```python
from build123d import *

# Parameters (mm, degrees)
SKETCH1_W              = 220
SKETCH1_H              = 225
BOSS_EXTRUDE1_DEPTH    = 16
CUT_EXTRUDE1_REACH     = 160.153
SKETCH2_R              = 4
CUT_EXTRUDE2_REACH     = 160.153
SKETCH3_W              = 12
SKETCH3_H              = 11.5
SKETCH4_R              = 8.5
CUT_EXTRUDE3_DEPTH     = 5
M10_TAPPED_HOLE2_D     = 8.5
M10_TAPPED_HOLE3_D     = 8.5
M10_TAPPED_HOLE4_D     = 8.5
CUT_EXTRUDE4_REACH     = 160.153
CUT_EXTRUDE6_REACH     = 160.153
F_10_0MM_DOWEL_HOLE1_D = 10
CUT_EXTRUDE7_REACH     = 160.153
SKETCH34_R             = 5


with BuildPart() as part:
    # Sketch1 → Boss-Extrude1 (new body)
    with BuildSketch(Plane(origin=(0, 0, 0), x_dir=(1, 0, 0), z_dir=(0, 1, 0))):
        Rectangle(SKETCH1_W, SKETCH1_H)
    extrude(amount=-BOSS_EXTRUDE1_DEPTH)

    # Sketch2 → Cut-Extrude1 (cut, up to next)
    with BuildSketch(Plane(origin=(0, 0, 0), x_dir=(1, 0, 0), z_dir=(0, 1, 0)), mode=Mode.PRIVATE) as cut_extrude1_sk1:
        with Locations(Location((-21.75, 10.23, 0), (0, 0, 270))):
            Circle(SKETCH2_R)
    cut_extrude1_tool1 = extrude(cut_extrude1_sk1.sketch, amount=-CUT_EXTRUDE1_REACH, mode=Mode.PRIVATE) & part.part
    add(cut_extrude1_tool1.solids().sort_by_distance((-21.75, 0, -10.23))[0], mode=Mode.SUBTRACT)

    # Sketch3 → Cut-Extrude2 (cut, up to next)
    with BuildSketch(Plane.XZ.offset(16), mode=Mode.PRIVATE) as cut_extrude2_sk1:
        with BuildLine():
            Line((-77.87, 101), (-67.87, 101))
            ThreePointArc((-67.87, 101), (-67.162893219, 101.292893219), (-66.87, 102))
            Line((-66.87, 102), (-66.87, 112.5))
            Line((-66.87, 112.5), (-78.87, 112.5))
            Line((-78.87, 112.5), (-78.87, 102))
            ThreePointArc((-78.87, 102), (-78.577106781, 101.292893219), (-77.87, 101))
        make_face()
    cut_extrude2_tool1 = extrude(cut_extrude2_sk1.sketch, amount=-CUT_EXTRUDE2_REACH, mode=Mode.PRIVATE) & part.part
    # Sketch3 → Cut-Extrude2 (cut, up to next)
    with BuildSketch(Plane.XZ.offset(16), mode=Mode.PRIVATE) as cut_extrude2_sk2:
        with Locations((3.38, 106.75)):
            Rectangle(SKETCH3_W, SKETCH3_H)
    cut_extrude2_tool2 = extrude(cut_extrude2_sk2.sketch, amount=-CUT_EXTRUDE2_REACH, mode=Mode.PRIVATE) & part.part
    add(cut_extrude2_tool1.solids().sort_by_distance((-72.87, -16, 106.767242))[0], mode=Mode.SUBTRACT)
    add(cut_extrude2_tool2.solids().sort_by_distance((3.38, -16, 106.75))[0], mode=Mode.SUBTRACT)

    # Sketch4 → Cut-Extrude3 (cut)
    with BuildSketch(Plane.XZ.offset(16)):
        with Locations(Location((-35, 100, 0), (0, 0, 270))):
            Circle(SKETCH4_R)
        with Locations(Location((25, 100, 0), (0, 0, 270))):
            Circle(SKETCH4_R)
        with Locations(Location((70, 100, 0), (0, 0, 270))):
            Circle(SKETCH4_R)
        with Locations(Location((-35, -100, 0), (0, 0, 270))):
            Circle(SKETCH4_R)
        with Locations(Location((25, -100, 0), (0, 0, 270))):
            Circle(SKETCH4_R)
        with Locations(Location((70, -100, 0), (0, 0, 270))):
            Circle(SKETCH4_R)
    extrude(amount=-CUT_EXTRUDE3_DEPTH, mode=Mode.SUBTRACT)

    # M10 Tapped Hole2 (through all)
    with Locations(Plane(origin=(0, 0, 0), x_dir=(1, 0, 0), z_dir=(0, 1, 0))):
        with Locations((-95, -67.5), (-95, -37.5), (-95, 0), (-95, 37.5), (-95, 67.5), (95, 67.5), (95, 37.5), (95, 0), (95, -37.5), (95, -67.5)):
            Hole(M10_TAPPED_HOLE2_D / 2)

    # M10 Tapped Hole3 (through all)
    with Locations(Plane(origin=(0, 0, 0), x_dir=(1, 0, 0), z_dir=(0, 1, 0))):
        with Locations((-56, 92.5), (-5, 92.5), (47.5, 92.5)):
            Hole(M10_TAPPED_HOLE3_D / 2)

    # M10 Tapped Hole4 (through all)
    with Locations(Plane(origin=(0, 0, 0), x_dir=(1, 0, 0), z_dir=(0, 1, 0))):
        with Locations((-13, -90.5), (47.5, -90.5), (-56, -90.5)):
            Hole(M10_TAPPED_HOLE4_D / 2)

    # Sketch24 → Cut-Extrude4 (cut, up to next)
    with BuildSketch(Plane(origin=(0, 0, 0), x_dir=(1, 0, 0), z_dir=(0, 1, 0)), mode=Mode.PRIVATE) as cut_extrude4_sk1:
        with BuildLine():
            Line((2.25, -35.27), (2.25, -71.53))
            ThreePointArc((2.25, -71.53), (1.371320344, -73.651320344), (-0.75, -74.53))
            Line((-0.75, -74.53), (-42.75, -74.53))
            ThreePointArc((-42.75, -74.53), (-44.871320344, -73.651320344), (-45.75, -71.53))
            Line((-45.75, -71.53), (-45.75, -35.27))
            ThreePointArc((-45.75, -35.27), (-44.871320344, -33.148679656), (-42.75, -32.27))
            Line((-42.75, -32.27), (-40.75, -32.27))
            Line((-40.75, -32.27), (-40.75, -38.4))
            ThreePointArc((-40.75, -38.4), (-38.992640687, -42.642640687), (-34.75, -44.4))
            Line((-34.75, -44.4), (-30.75, -44.4))
            ThreePointArc((-30.75, -44.4), (-28.628679656, -45.278679656), (-27.75, -47.4))
            Line((-27.75, -47.4), (-27.75, -63.53))
            ThreePointArc((-27.75, -63.53), (-21.75, -69.53), (-15.75, -63.53))
            Line((-15.75, -63.53), (-15.75, -47.4))
            ThreePointArc((-15.75, -47.4), (-14.871320344, -45.278679656), (-12.75, -44.4))
            Line((-12.75, -44.4), (-8.75, -44.4))
            ThreePointArc((-8.75, -44.4), (-4.507359313, -42.642640687), (-2.75, -38.4))
            Line((-2.75, -38.4), (-2.75, -32.27))
            Line((-2.75, -32.27), (-0.75, -32.27))
            ThreePointArc((-0.75, -32.27), (1.371320344, -33.148679656), (2.25, -35.27))
        make_face()
    cut_extrude4_tool1 = extrude(cut_extrude4_sk1.sketch, amount=-CUT_EXTRUDE4_REACH, mode=Mode.PRIVATE) & part.part
    add(cut_extrude4_tool1.solids().sort_by_distance((-15.110476, 0, 55.465))[0], mode=Mode.SUBTRACT)

    # Sketch29 → Cut-Extrude6 (cut, up to next)
    with BuildSketch(Plane.XZ.offset(16), mode=Mode.PRIVATE) as cut_extrude6_sk1:
        with BuildLine():
            Line((-2.75, -47.73), (-0.75, -47.73))
            ThreePointArc((-0.75, -47.73), (1.371320344, -48.608679656), (2.25, -50.73))
            Line((2.25, -50.73), (2.25, -71.53))
            ThreePointArc((2.25, -71.53), (1.371320344, -73.651320344), (-0.75, -74.53))
            Line((-0.75, -74.53), (-42.75, -74.53))
            ThreePointArc((-42.75, -74.53), (-44.871320344, -73.651320344), (-45.75, -71.53))
            Line((-45.75, -71.53), (-45.75, -50.73))
            ThreePointArc((-45.75, -50.73), (-44.871320344, -48.608679656), (-42.75, -47.73))
            Line((-42.75, -47.73), (-40.75, -47.73))
            Line((-40.75, -47.73), (-40.75, -69.53))
            Line((-40.75, -69.53), (-2.75, -69.53))
            Line((-2.75, -69.53), (-2.75, -47.73))
        make_face()
    cut_extrude6_tool1 = extrude(cut_extrude6_sk1.sketch, amount=-CUT_EXTRUDE6_REACH, mode=Mode.PRIVATE) & part.part
    add(cut_extrude6_tool1.solids().sort_by_distance((-1.75, -16, -48.279749))[0], mode=Mode.SUBTRACT)

    # Ø10.0mm Dowel Hole1 (through all)
    with Locations(Plane(origin=(0, 0, 0), x_dir=(1, 0, 0), z_dir=(0, 1, 0))):
        with Locations((54.5, -63.53), (67.5, -38.4), (41.5, -38.4), (19.38, 26.73), (19.38, -6.27)):
            Hole(F_10_0MM_DOWEL_HOLE1_D / 2)

    # Sketch34 → Cut-Extrude7 (cut, up to next)
    with BuildSketch(Plane(origin=(0, 0, 0), x_dir=(1, 0, 0), z_dir=(0, 1, 0)), mode=Mode.PRIVATE) as cut_extrude7_sk1:
        with Locations(Location((54.5, 10.23, 0), (0, 0, 270))):
            Circle(SKETCH34_R)
    cut_extrude7_tool1 = extrude(cut_extrude7_sk1.sketch, amount=-CUT_EXTRUDE7_REACH, mode=Mode.PRIVATE) & part.part
    add(cut_extrude7_tool1.solids().sort_by_distance((54.5, 0, -10.23))[0], mode=Mode.SUBTRACT)

    # Cut-Sweep1: sweep along a curve in space
    with BuildLine() as cut_sweep1_path:
        ThreePointArc((54.5, 0, -5.23), (58.035533906, 0, -6.694466094), (59.5, 0, -10.23))
        ThreePointArc((59.5, 0, -10.23), (58.035533906, 0, -13.765533906), (54.5, 0, -15.23))
        ThreePointArc((54.5, 0, -15.23), (50.964466094, 0, -13.765533906), (49.5, 0, -10.23))
        ThreePointArc((49.5, 0, -10.23), (50.964466094, 0, -6.694466094), (54.5, 0, -5.23))
    # Sketch35 → Cut-Sweep1 (sweep, cut)
    with BuildSketch(Plane.XY.offset(-10.23)):
        Polygon((59.5, -10), (60.024077793, 0), (59.5, 0), align=None)
    sweep(path=cut_sweep1_path.line, mode=Mode.SUBTRACT)


solid = part.part
```
Design review of the part built by this model. Coordinates are the model's own, in mm. A direction names the side the tool comes from. Coordinates: 2 decimals unless noted, no trailing zeros. Loops run counter-clockwise (first coordinate to the right, second up) from the corner with the lowest first, then second, coordinate; pieces in that order, holes last.
Q1. We need section D-D on y = -2.5. State how many separate pieces and enclosed holes the cut face has, and give its area (3 significant figures).
Reported:
separate pieces: 1
enclosed holes: 25
area: 46,000 mm2
Q2. We need section B-B on z = -37.5. State the section outline as (x, y) points.
Reported:
outline: (-110, -16) - (-99.25, -16) - (-99.25, 0) - (-110, 0) - close; (-90.75, -16) - (90.75, -16) - (90.75, 0) - (-90.75, 0) - close; (99.25, -16) - (110, -16) - (110, 0) - (99.25, 0) - close
Q3. For pin 1 (13.5 mm diameter, centred on x = 70, z = 100, fed in from -Y); pin 2 (5 mm diameter, centred on x = -74, y = -6.5, fed in from +Z); pin 3 (10 mm diameter, centred on x = -95, z = -67.5, fed in from -Y), all flat-tipped, find the tip position at first contact; note any pin that passes through.
Reported:
pin 1: stops at y = -11
pin 2: stops at z = 101
pin 3: stops at y = -16
Q4. The part is to be moulded in two halves that separate along X. For faces 1 (the face through (-110, -8, 2)), 2 (the face through (-2, 0, -2)), 3 (the face through (99.246, -8.112, -37.687)), say which applies: +X half, -X half, draft (parallel to the pull), parting line (faces both ways), or undercut.
Reported:
face 1: -X half
face 2: draft
face 3: undercut
Q5. We need section C-C on x = 29. State the section outline as (y, z) points, and give its area (3 significant figures).
Reported:
outline: (-16, -112.5) - (0, -112.5) - (0, 112.5) - (-16, 112.5) - (-16, 107.5) - (-11, 107.5) - (-11, 92.5) - (-16, 92.5) - (-16, -92.5) - (-11, -92.5) - (-11, -107.5) - (-16, -107.5) - close
area: 3,450 mm2
Q6. Tool access review of faces 4 (the face through (75.745, -13.535, 106.265)), 5 (the face through (-22, -8, -69.53)), 6 (the face through (-66.87, -8, 107)): name each direction out of +Z, -Z, +X, -X, +Y, -Y from which nothing blocks a thin tool from reaching the whole face with its end or side.
Reported:
face 4: -Y
face 5: +Y, -Y
face 6: +Z, +Y, -Y
Q7. To check wall thickness, follow line 1 (X direction, y = -1, z = -0.5); line 2 (Z direction, x = 47.5, y = -7.75); line 3 (X direction, y = -13.65, z = 100). State the ranges of each line that lie inside material, in increasing order.
Reported:
line 1: x = -110 to -99.22, -90.78 to 90.78, 99.22 to 110
line 2: z = -112.5 to -96.75, -88.25 to 86.25, 94.75 to 112.5
line 3: x = -110 to -43.5, -26.5 to 16.5, 33.5 to 61.5, 78.5 to 110
Q8. We need section A-A on x = -56. State the section outline as (y, z) points, and give its area (3 significant figures).
Reported:
outline: (-16, -112.5) - (0, -112.5) - (0, -96.75) - (-16, -96.75) - close; (-16, -88.25) - (0, -88.25) - (0, 86.25) - (-16, 86.25) - close; (-16, 94.75) - (0, 94.75) - (0, 112.5) - (-16, 112.5) - close
area: 3,330 mm2
